CAD build for the part. Positions are in the model's coordinates, mm. Face numbers are marked on the shaded views. A direction names the side the tool comes from. Coordinates: 2 decimals unless noted, no trailing zeros. Loops run counter-clockwise (first coordinate to the right, second up) from the corner with the lowest first, then second, coordinate; pieces in that order, holes last. Notation, with made-up numbers: (-29.75, -30.5) -> (-10.75, -30.5) arc R21 ccw to (-10.75, 2.5) -> close; hole circle Ø10 at (46.25, 8). An arc over 180 degrees is marked (long way). Write item = value, one per line. Start each with the question number.
(1) Flat gauge pins, fed straight in: P1, Ø6.5, axis at x = 83.5, z = -16, coming from the +Y side; P2, Ø1.2, axis at x = 88.5, y = 1, coming from the -Z side; P3, Ø0.9, axis at x = 82.5, z = 12.5, coming from the +Y side. Where does each tip first touch, or does it go through?
(2) Band-saw the part on A-A (x = -32.5). Write the cut outline in (y, z), and give its area (3 significant figures).
(3) Drill centre lines: line 1 (X direction, y = 5, z = -26); line 2 (Y direction, x = 80.5, z = 39.5); line 3 (X direction, y = 6.5, z = 7). Where is each one in solid material? Low to high. Write a range as from..to.
(4) Tool access for the marked faces 1, 2, 3 and 4: list every direction of +Z, -Z, +X, -X, +Y, -Y with a clear straight run to the whole face (end or side of a thin tool).
```python
from build123d import *

# Parameters (mm, degrees)
SKETCH_2_W          = 180
SKETCH_2_H          = 94
EXTRUDE_1_DEPTH     = 1.5
CUT_EXTRUDE_1_DEPTH = 1.5
FILLET_1_R          = 1
SKETCH_4_W          = 17
SKETCH_4_H          = 68
EXTRUDE_2_DEPTH     = 15
SKETCH_6_W          = 14
SKETCH_6_H          = 8
CUT_EXTRUDE_3_DEPTH = 7
SKETCH_7_R          = 1.5
CUT_EXTRUDE_4_DEPTH = 8
SKETCH_5_R          = 1.5
CUT_EXTRUDE_2_DEPTH = 103.635276587


with BuildPart() as part:
    # 草图2 → 凸台-拉伸1 (new body)
    with BuildSketch(Plane(origin=(0, 0, 0), x_dir=(1, 0, 0), z_dir=(0, 1, 0))):
        Rectangle(SKETCH_2_W, SKETCH_2_H)
    extrude(amount=EXTRUDE_1_DEPTH)

    # 草图3 → 切除-拉伸1 (cut)
    with BuildSketch(Plane(origin=(0, 1.5, 0), x_dir=(1, 0, 0), z_dir=(0, 1, 0))):
        with BuildLine():
            Line((85, 47), (85, 40))
            ThreePointArc((85, 40), (85.585786438, 38.585786438), (87, 38))
            Line((87, 38), (90, 38))
            Line((90, 38), (90, 47))
            Line((90, 47), (85, 47))
        make_face()
        with BuildLine():
            Line((87, -38), (90, -38))
            Line((90, -38), (90, -47))
            Line((90, -47), (85, -47))
            Line((85, -47), (85, -40))
            ThreePointArc((85, -40), (85.585786438, -38.585786438), (87, -38))
        make_face()
        with BuildLine():
            Line((-90, -47), (-90, -38))
            Line((-90, -38), (-87, -38))
            ThreePointArc((-87, -38), (-85.585786438, -38.585786438), (-85, -40))
            Line((-85, -40), (-85, -47))
            Line((-85, -47), (-90, -47))
        make_face()
        with BuildLine():
            Line((-90, 47), (-90, 38))
            Line((-90, 38), (-87, 38))
            ThreePointArc((-87, 38), (-85.585786438, 38.585786438), (-85, 40))
            Line((-85, 40), (-85, 47))
            Line((-85, 47), (-90, 47))
        make_face()
    extrude(amount=-CUT_EXTRUDE_1_DEPTH, mode=Mode.SUBTRACT)

    # 圆角1
    fillet_1_edges = [part.edges().sort_by_distance(p)[0] for p in [
        (85, 0.75, -47),
        (90, 0.75, -38),
        (90, 0.75, 38),
        (85, 0.75, 47),
        (-85, 0.75, 47),
        (-90, 0.75, 38),
        (-90, 0.75, -38),
        (-85, 0.75, -47),
    ]]
    fillet(fillet_1_edges, radius=FILLET_1_R)

    # 草图4 → 凸台-拉伸2 (add)
    with BuildSketch(Plane(origin=(0, 1.5, 0), x_dir=(1, 0, 0), z_dir=(0, 1, 0))):
        with Locations((81, -2.5)):
            Rectangle(SKETCH_4_W, SKETCH_4_H)
    extrude(amount=EXTRUDE_2_DEPTH)

    # 草图6 → 切除-拉伸3 (cut)
    with BuildSketch(Plane(origin=(0, 16.5, 0), x_dir=(1, 0, 0), z_dir=(0, 1, 0))):
        with Locations((82.5, 26)):
            Rectangle(SKETCH_6_W, SKETCH_6_H)
        with Locations((82.5, 16.5)):
            Rectangle(SKETCH_6_W, SKETCH_6_H)
        with Locations((82.5, 7)):
            Rectangle(SKETCH_6_W, SKETCH_6_H)
        with Locations((82.5, -2.5)):
            Rectangle(SKETCH_6_W, SKETCH_6_H)
        with Locations((82.5, -12)):
            Rectangle(SKETCH_6_W, SKETCH_6_H)
        with Locations((82.5, -21.5)):
            Rectangle(SKETCH_6_W, SKETCH_6_H)
        with Locations((82.5, -31)):
            Rectangle(SKETCH_6_W, SKETCH_6_H)
    extrude(amount=-CUT_EXTRUDE_3_DEPTH, mode=Mode.SUBTRACT)

    # 草图7 → 切除-拉伸4 (cut)
    with BuildSketch(Plane(origin=(0, 9.5, 0), x_dir=(1, 0, 0), z_dir=(0, 1, 0))):
        with Locations(Location((82.5, 26, 0), (0, 0, 270))):
            Circle(SKETCH_7_R)
        with Locations(Location((82.5, 16.5, 0), (0, 0, 270))):
            Circle(SKETCH_7_R)
        with Locations(Location((82.5, 7, 0), (0, 0, 270))):
            Circle(SKETCH_7_R)
        with Locations(Location((82.5, -2.5, 0), (0, 0, 270))):
            Circle(SKETCH_7_R)
        with Locations(Location((82.5, -12, 0), (0, 0, 270))):
            Circle(SKETCH_7_R)
        with Locations(Location((82.5, -21.5, 0), (0, 0, 270))):
            Circle(SKETCH_7_R)
        with Locations(Location((82.5, -31, 0), (0, 0, 270))):
            Circle(SKETCH_7_R)
    extrude(amount=-CUT_EXTRUDE_4_DEPTH, mode=Mode.SUBTRACT)

    # 草图5 → 切除-拉伸2 (cut, through all)
    with BuildSketch(Plane(origin=(0, 1.5, 0), x_dir=(1, 0, 0), z_dir=(0, 1, 0))):
        with Locations(Location((76, -43, 0), (0, 0, 270))):
            Circle(SKETCH_5_R)
    extrude(amount=-CUT_EXTRUDE_2_DEPTH, mode=Mode.SUBTRACT)


solid = part.part
```
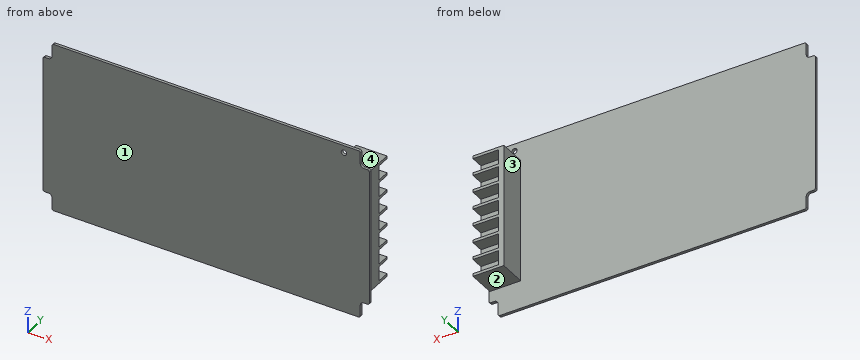
Findings below:
q1.P1 = 9.5
q1.P2 = -38
q1.P3 = 1.5
q2.outline = (0, -47) -> (1.5, -47) -> (1.5, 47) -> (0, 47) -> close
q2.area = 141 mm²
q3.line_1 = 72.5..81, 84..89.5
q3.line_2 = 0..1.5
q3.line_3 = 72.5..89.5
q4.face_1 = +Z, -Z, +X, -X, -Y
q4.face_2 = -Z, +X, -X, +Y
q4.face_3 = +Z, -Z, -X, +Y
q4.face_4 = +Z, +X, -X, +Y
